```python
from build123d import *

# Parameters (mm, degrees)
F2_R     = 4.7625
F3_DEPTH = 19.05


with BuildPart() as f3:
    # F2 (on Right) → F3 (new body)
    with BuildSketch(Plane.YZ):
        with BuildLine():
            ThreePointArc((-1015.907792, 792.417112), (-1036.686006, 818.394405), (-1065.357711, 801.527653))
            Line((-1065.357711, 801.527653), (-1110.364914, 667.998314))
            Line((-1110.364914, 667.998314), (-1314.37809, 312.639923))
            ThreePointArc((-1314.37809, 312.639923), (-1306.780078, 282.66374), (-1276.576197, 289.299018))
            Line((-1276.576197, 289.299018), (-1020.491481, 675.813437))
            Line((-1020.491481, 675.813437), (-1015.907792, 792.417112))
        make_face()
        with Locations((-1295.10365, 301.574363)):
            Circle(F2_R, mode=Mode.SUBTRACT)
        with Locations((-1037.116024, 677.367714)):
            Circle(F2_R, mode=Mode.SUBTRACT)
        with Locations((-1041.288189, 793.414815)):
            Circle(F2_R, mode=Mode.SUBTRACT)
    extrude(amount=F3_DEPTH)


solid = f3.part
```
Geometry: final body of the model. Coordinates: model frame, mm. Give positions to 0.01 mm unless a question says otherwise; leave off trailing zeros. Order: outer loops, then holes, each group sorted by start corner. A loop starts at its lowest first (then second) coordinate and runs counter-clockwise, first axis right, second up. Notation, with made-up numbers: (-8, 14) -> (23, 14) arc R19 cw to (23, 45) -> close; hole circle Ø7 at (-14, 49). An arc over 180 degrees is marked (long way). Write each question's results on one line, items separated by ' | '. Start each with the question number.
1) Section C-C (z = 462.5). Return loops of the section in (x, y).
2) Section B-B (y = -1201). Return loops of the section in (x, z).
3) First-contact query: pin 1 (1 mm diameter, centred on x = 2.5, y = -1183.5, fed in from -Z); pin 2 (6 mm diameter, centred on x = 13, z = 392, fed in from -Y); pin 3 (5 mm diameter, centred on x = 8, y = -1054, fed in from -Z). Flat tips, straight axial feed; report the tip coordinate or a pass-through.
4) Section A-A (x = 14.5). Count the separate pieces of the cut face and the enclosed holes in it, then the cut area to 3 significant figures.
5) Line query: line 1 (Y direction, x = 4, z = 676); line 2 (Z direction, x = 18.25, y = -1044.5); line 3 (Y direction, x = 9.25, z = 335). Output: solid intervals per line, ascending. Write a range as from..to.
6) Draft query along Z for faces 1 (the flat face through (19.05, -1156, 550)), 2 (the flat face through (9.39, -1018.23, 733.3)), 3 (the cylindrical face through (9.39, -1292.54, 305.59)). Return one class per face: pulls with the +Z half, pulls with the -Z half, needs draft (parallel to the pull), parting line crosses it, or undercut.
Calculated:
1) outline: (0, -1228.34) -> (19.05, -1228.34) -> (19.05, -1161.82) -> (0, -1161.82) -> close
2) outline: (0, 403.37) -> (19.05, 403.37) -> (19.05, 510.13) -> (0, 510.13) -> close
3) pin 1: z = 429.03 | pin 2: y = -1270.54 | pin 3: z = 621.46
4) separate pieces: 1 | enclosed holes: 3 | area: 35,600 mm2
5) line 1: -1107.67..-1041.68, -1032.55..-1020.48 | line 2: 639.58..789.9, 796.93..818.61 | line 3: -1301.54..-1246.3
6) face 1: needs draft | face 2: pulls with the -Z half | face 3: undercut
